from build123d import *

# Parameters (mm, degrees)
CHAMFER_1_SIZE = 0.5


with BuildPart() as part:
    # Sketch 1 → Revolve 1 (revolve)
    with BuildSketch(Plane.XY, mode=Mode.PRIVATE) as revolve_1_sk:
        Polygon((-26, 28), (-26, 11), (-6.947441117, 0), (-3, 0), (-3, 6), (-11.509618943, 6), (-24.5, 13.5), (-24.5, 16), (-23, 16), (-23, 28), align=None)
    revolve(revolve_1_sk.sketch.rotate(Axis((0, 26.168985987, 0), (0, -1, 0)), 270), axis=Axis((0, 26.168985987, 0), (0, -1, 0)))

    # Chamfer 1
    chamfer_1_edges = [part.edges().sort_by_distance(p)[0] for p in [
        (0, 0, -3),
        (0, 28, -26),
        (0, 28, -23),
    ]]
    chamfer(chamfer_1_edges, length=CHAMFER_1_SIZE)


solid = part.part
Model file for the job. Use its own axes, mm. A direction names the side the tool comes from. Give positions to 0.01 mm unless a question says otherwise; leave off trailing zeros. Loops run counter-clockwise (first coordinate to the right, second up) from the corner with the lowest first, then second, coordinate; pieces in that order, holes last. Notation, with made-up numbers: (71.25, 44) - (107.25, 44) arc R27 cw to (107.25, 79) - close; hole circle Ø1 at (8.25, -35.75). An arc over 180 degrees is marked (long way). Use one line per item in the form item = value.
(1) Cut at A-A (z = 0). Give the cut face in (x, y).
Determined:
outline = (-26, 11) - (-6.95, 0) - (-3.5, 0) - (-3, 0.5) - (-3, 6) - (-11.51, 6) - (-24.5, 13.5) - (-24.5, 16) - (-23, 16) - (-23, 27.5) - (-23.5, 28) - (-25.5, 28) - (-26, 27.5) - close; (3, 0.5) - (3.5, 0) - (6.95, 0) - (26, 11) - (26, 27.5) - (25.5, 28) - (23.5, 28) - (23, 27.5) - (23, 16) - (24.5, 16) - (24.5, 13.5) - (11.51, 6) - (3, 6) - close
(2) Cut at B-B (x = 0). Give the cut face in (y, z), then the cut area to 3 significant figures.
Determined:
outline = (0, -6.95) - (11, -26) - (27.5, -26) - (28, -25.5) - (28, -23.5) - (27.5, -23) - (16, -23) - (16, -24.5) - (13.5, -24.5) - (6, -11.51) - (6, -3) - (0.5, -3) - (0, -3.5) - close; (0, 3.5) - (0.5, 3) - (6, 3) - (6, 11.51) - (13.5, 24.5) - (16, 24.5) - (16, 23) - (27.5, 23) - (28, 23.5) - (28, 25.5) - (27.5, 26) - (11, 26) - (0, 6.95) - close
area = 265 mm^2
(3) 3-axis set-ups, long thin cutter, end or side, ignore diameter. For faces 1 (the face through (2.4, 6, -2.4)), 2 (the face through (4.79, 0.534, -6.247)): which of +Z, -Z, +X, -X, +Y, -Y reach the whole face in a straight line?
Determined:
face_1 = +Y
face_2 = -Y
(4) Cut at C-C (y = 18.5). Give the cut face in (x, z), then the cut area to 3 significant figures.
Determined:
outline = circle Ø52 at (0, 0); hole circle Ø46 at (0, 0)
area = 462 mm^2
(5) Pull direction Y, two halves, no side cores. Call faces 3 (the face through (3, 0, 3)), 4 (the face through (11, 28, -21)), 5 (the face through (-7.36, 14.77, 23.37)): pulls with the +Y half, pulls with the -Y half, needs draft (parallel to the pull), parting line crosses it, or undercut.
Determined:
face_3 = pulls with the -Y half
face_4 = pulls with the +Y half
face_5 = undercut
(6) Drop flat-ended pins along their axis: P1, Ø12, axis at y = 9.5, z = 12, coming from the +X side; P2, Ø6, axis at y = 7.5, z = 3.5, coming from the -X side; P3, Ø10, axis at y = 8.5, z = 16.5, coming from the -X side. Give the stop position or say it passes through.
Determined:
P1 = 25.25
P2 = -24.9
P3 = -22.98
(7) Drill centre lines: L1, parallel to X at y = 14.65, z = 0; L2, parallel to X at y = 22, z = 0; L3, parallel to Y at x = 6, z = -23.5. Where is each one in solid material? Low to high.
Determined:
L1 = -26 to -24.5, 24.5 to 26
L2 = -26 to -23, 23 to 26
L3 = 9.99 to 13.36, 16 to 28
